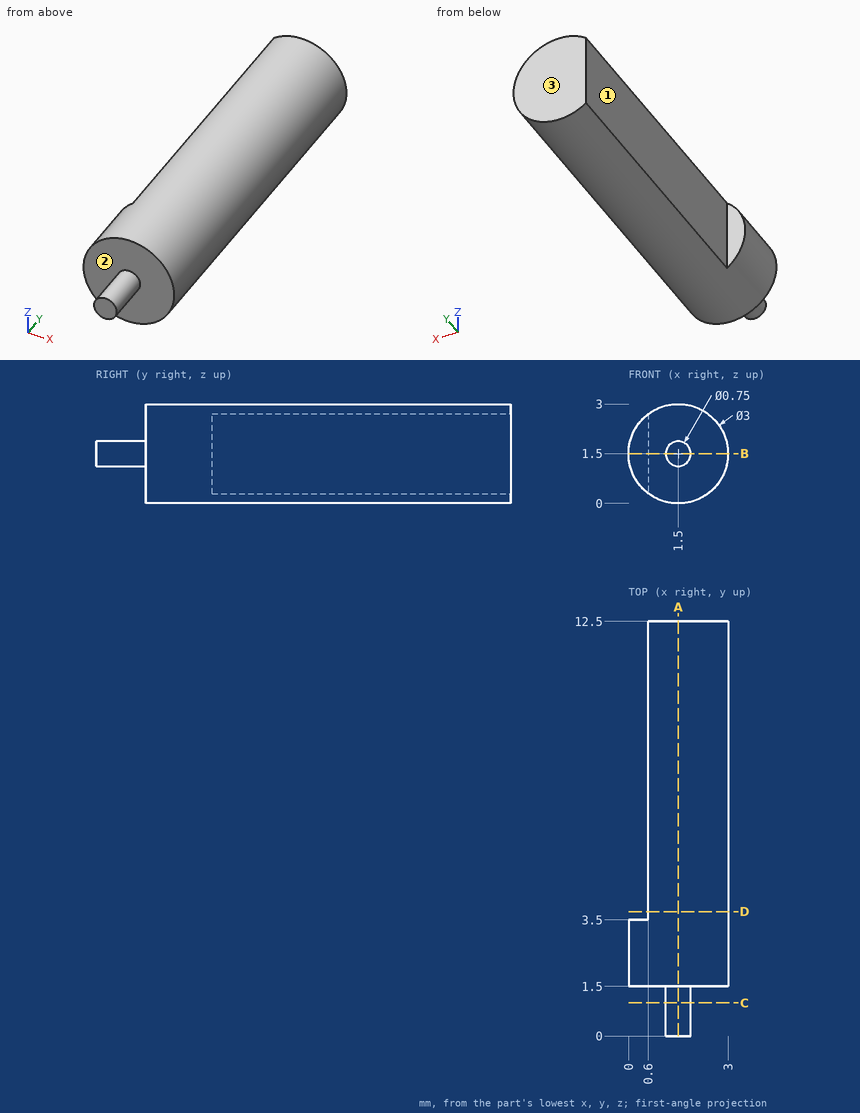
Here's the drawing with two shaded views (mm, measured from the low corner). I have some questions. A direction names the side the tool comes from. Coordinates: 2 decimals unless noted, no trailing zeros. Write each loop counter-clockwise with the first axis right and the second up, starting at its lowest first coordinate (ties: lowest second). Pieces come first, ordered by that corner, then holes. Notation, with made-up numbers: (57, 65) -> (86, 65) arc R15 cw to (86, 75) -> close; hole circle Ø9 at (70, 21.25). An arc over 180 degrees is marked (long way). Use a Markdown table: item, result. Add a question column.
(1) Please list where these lines run through material, in increasing order: line 1 (Y direction, x = 0.9, z = 2.6); line 2 (Z direction, x = 1.6, y = 3.25); line 3 (Y direction, x = 0.2, z = 0.9).
(2) If we section it at B-B, the plane z = 1.5: Write out the boundary of the cut face in (x, y) (3 decimals), and give its area (3 significant figures).
(3) If we section it at A-A, the plane x = 1.5: Write out the boundary of the cut face in (y, z) (3 decimals).
(4) If we section it at C-C, the plane y = 1: Write out the boundary of the cut face in (x, z) (3 decimals), and give its area (3 significant figures).
(5) I'm going to push flat-ended pins straight in: P1, Ø1.5, axis at y = 9, z = 2, coming from the -X side; P2, Ø1.5, axis at x = 2.5, y = 3, coming from the -Z side; P3, Ø0.9, axis at x = 1.5, z = 1.5, coming from the -Y side. Where does each tip first touch, or does it pass through?
(6) If we section it at D-D, the plane y = 3.75: Write out the boundary of the cut face in (x, z).
(7) For the marked faces 1, 2 and 3, which set-ups out of +Z, -Z, +X, -X, +Y, -Y let a thin tool reach every point of the face, with its end or its side?
Outcome:
| question | item | result |
|---|---|---|
| 1 | line 1 | y = 1.5 to 12.5 |
| 1 | line 2 | z = 0 to 3 |
| 1 | line 3 | y = 1.5 to 3.5 |
| 2 | outline | (0, 1.5) -> (1.125, 1.5) -> (1.125, 0) -> (1.875, 0) -> (1.875, 1.5) -> (3, 1.5) -> (3, 12.5) -> (0.6, 12.5) -> (0.6, 3.5) -> (0, 3.5) -> close |
| 2 | area | 28.7 mm^2 |
| 3 | outline | (0, 1.125) -> (1.5, 1.125) -> (1.5, 0) -> (12.5, 0) -> (12.5, 3) -> (1.5, 3) -> (1.5, 1.875) -> (0, 1.875) -> close |
| 4 | outline | circle Ø0.75 at (1.5, 1.5) |
| 4 | area | 0.442 mm^2 |
| 5 | P1 | stops at x = 0.6 |
| 5 | P2 | stops at z = 0.02 |
| 5 | P3 | stops at y = 0 |
| 6 | outline | (0.6, 0.3) arc R1.5 ccw (long way) to (0.6, 2.7) -> close |
| 7 | face 1 | +Z, -Z, -X, +Y |
| 7 | face 2 | -Y |
| 7 | face 3 | +Z, -Z, +X, -X, +Y |
